Source: CAD feature listing. Evaluate the final solid. Frame: model axes, mm. A direction names the side the tool comes from. Round coordinates to 2 decimals unless told otherwise and drop trailing zeros. Loops run counter-clockwise (first coordinate to the right, second up) from the corner with the lowest first, then second, coordinate; pieces in that order, holes last.
(1) First-contact query: pin 1 Ø3 at (x, y) = (4, -37.5) entering from -Z; pin 2 Ø4 at (x, y) = (3.5, -43) entering from -Z. Flat tips, straight axial feed; report the tip coordinate or a pass-through.
(2) Section A-A, the plane x = 6.75. Return the cut outline in (y, z), plus the area to 3 significant figures.
(3) Section B-B, the plane y = -47.25. Return the cut outline in (x, z), plus the area to 3 significant figures.
(4) Section D-D, the plane y = -43. Return the cut outline in (x, z).
(5) Set-up query: faces 1 (the flat face through (4, -33.541, 22)), 2 (the flat face through (4, -37, -15.24)). Return all of +Z, -Z, +X, -X, +Y, -Y with unobstructed straight access to the full face (end or side cutting, diameter ignored); none if empty.
(6) Section C-C, the plane x = 3.25. Return the cut outline in (y, z).
(7) Material intervals for probe 1 along Y at (x, z) = (5.25, -15.5); probe 2 along Z at (x, y) = (5.5, -36); probe 3 along Z at (x, y) = (2.25, -47.25), sorted ascending.
```python
from build123d import *

# Parameters (mm, degrees)
F1_DEPTH = 7.62
F3_DEPTH = 25.4


with BuildPart() as f1:
    # F0 (on Right) → F1 (new body)
    with BuildSketch(Plane.YZ):
        Polygon((-33.541034, 60.960074), (-48.781034, 60.960074), (-48.781034, -15.239926), (-42.431034, -15.239926), (-39.891034, -15.239926), (-33.541034, -15.239926), align=None)
        with BuildLine():
            Line((-42.431034, -15.239926), (-48.781034, -15.239926))
            ThreePointArc((-48.781034, -15.239926), (-46.729882, -22.645235), (-41.161034, -27.939926))
            ThreePointArc((-41.161034, -27.939926), (-40.516197, -27.574381), (-39.891034, -27.176124))
            Line((-39.891034, -27.176124), (-39.891034, -15.239926))
            Line((-39.891034, -15.239926), (-42.431034, -15.239926))
        make_face()
    extrude(amount=F1_DEPTH)

    # F2 (on face) → F3 (cut)
    with BuildSketch(Plane(origin=(0, -33.541034, 0), x_dir=(-1, 0, 0), z_dir=(0, 1, 0))):
        with BuildLine():
            ThreePointArc((0, -27.939926), (-5.568848, -22.645235), (-7.62, -15.239926))
            Line((-7.62, -15.239926), (-7.62, -27.939926))
            Line((-7.62, -27.939926), (0, -27.939926))
        make_face()
    extrude(amount=-F3_DEPTH, mode=Mode.SUBTRACT)


solid = f1.part
```
Output values:
1. pin 1: stops at z = -15.24
1. pin 2: stops at z = -27
2. outline: (-48.78, -15.24) arc R14.39 ccw to (-47.91, -20.17) - (-39.89, -20.17) - (-39.89, -15.24) - (-33.54, -15.24) - (-33.54, 60.96) - (-48.78, 60.96) - close
2. area: 1,200 mm2
3. outline: (0, -21.7) - (6.09, -21.7) arc R14.39 ccw to (7.62, -15.24) - (7.62, 60.96) - (0, 60.96) - close
3. area: 627 mm2
4. outline: (0, -26.77) - (1.84, -26.77) arc R14.39 ccw to (7.62, -15.24) - (7.62, 60.96) - (0, 60.96) - close
5. face 1: +Z, -Z, +X, -X, +Y
5. face 2: -Z, +X, -X, +Y
6. outline: (-48.78, -15.24) arc R14.39 ccw to (-44.41, -25.57) - (-39.89, -25.57) - (-39.89, -15.24) - (-33.54, -15.24) - (-33.54, 60.96) - (-48.78, 60.96) - close
7. probe 1: y = -48.78 to -39.89
7. probe 2: z = -15.24 to 60.96
7. probe 3: z = -21.7 to 60.96
